Check sheet for the modelled part. Datum: model origin and axes. Units: mm. A direction names the side the tool comes from. Round coordinates to 2 decimals unless told otherwise and drop trailing zeros. Put each result on its own line as item: value.
```python
from build123d import *

# Parameters (mm, degrees)
F1_DEPTH       = 72.5
F3_D           = 5
F3_CBORE_D     = 10
F3_CBORE_DEPTH = 5
F4_R           = 2.5
F5_R           = 2.5


# Not quite as in the source:
# - ends of sketch curves that miss each other by under 0.0002 mm in the source are joined
# - the dataset's text gives a spline's control points without its knots; the knots are read off the source's solid


with BuildPart() as f1:
    # F0 (on Front) → F1 (new body)
    with BuildSketch(Plane.XZ):
        with BuildLine():
            add(Edge.make_bspline(
                [(-56.5881601574, 0.0419234738), (-55.5197950815, -0.7442946781), (-53.1301338185, -2.2933127374), (-48.9084685045, -4.5561843947), (-44.1859500973, -6.7339324001), (-39.1068883918, -8.7916644331), (-33.8193544964, -10.6897211609), (-29.3644227389, -12.1035605133), (-25.8455914341, -13.1126993817), (-22.383504382, -14.0327971877), (-19.4313477815, -14.7259719893), (-17.3706943762, -15.160741157), (-16.9593766332, -15.2455717325)],
                knots=[0, 0, 0, 0, 0.03125, 0.0625, 0.09375, 0.125, 0.15625, 0.1875, 0.203125, 0.21875, 0.25, 0.2578399244, 0.2578399244, 0.2578399244, 0.2578399244], degree=3))
            add(Edge.make_bspline(
                [(-56.5881601574, 0.0419234738), (-55.5355017666, 0.8486239051), (-53.1764131036, 2.443347048), (-48.9992069483, 4.7861572474), (-44.3187202519, 7.053077305), (-39.2793074327, 9.2063486815), (-34.0283660726, 11.2037109249), (-29.6007919855, 12.7012369201), (-26.1016179695, 13.7765699234), (-22.65755408, 14.761891198), (-19.6168305087, 15.5368665147), (-17.4672919643, 16.0305431026), (-16.9593493648, 16.1441983995)],
                knots=[1.43705e-05, 1.43705e-05, 1.43705e-05, 1.43705e-05, 0.03125, 0.0625, 0.09375, 0.125, 0.15625, 0.1875, 0.203125, 0.21875, 0.25, 0.2597438328, 0.2597438328, 0.2597438328, 0.2597438328], degree=3))
            Line((-16.9593493648, 16.1441983995), (-16.9593493648, 38.671177907))
            Line((-16.9593493648, 38.671177907), (-76.9551545382, 38.671177907))
            Line((-76.9551545382, 38.671177907), (-76.9551545382, -38.248822093))
            Line((-76.9551545382, -38.248822093), (-16.9593493648, -38.248822093))
            Line((-16.9593493648, -38.248822093), (-16.9593766332, -15.2455717325))
        make_face()
    extrude(amount=F1_DEPTH)

    # F3 (through all)
    with Locations(Plane(origin=(-76.9551545382, 0, 0), x_dir=(0, -1, 0), z_dir=(-1, 0, 0))):
        with Locations((10, 28.671177907), (62.5, 28.671177907), (62.5, -28.248822093), (10, -28.248822093)):
            CounterBoreHole(F3_D / 2, F3_CBORE_D / 2, F3_CBORE_DEPTH)

    # F4
    f4_edges = [f1.edges().sort_by_distance(p)[0] for p in [
        (-76.955155, -72.5, 0.211178),
        (-76.955155, -36.25, 38.671178),
        (-76.955155, 0, 0.211178),
        (-76.955155, -36.25, -38.248822),
    ]]
    fillet(f4_edges, radius=F4_R)

    # F5
    f5_edges = [f1.edges().sort_by_distance(p)[0] for p in [
        (-16.959349, -36.25, 38.671178),
        (-16.959349, -72.5, 27.407688),
        (-16.959349, 0, 27.407688),
        (-16.959363, 0, -26.747197),
        (-16.959349, -36.25, -38.248822),
        (-16.959363, -72.5, -26.747197),
    ]]
    fillet(f5_edges, radius=F5_R)


solid = f1.part
```
Item 1: Release check for a two-part mould opening along Z. For faces 3 (the flat face through (-47, -36, -38.249)), 4 (the cylindrical face through (-76.24, -36.76, 37.92)), 5 (the cylindrical face through (-74.49, -58.53, 25.63)), 6 (the flat face through (-47, 0, 9)) record: +Z half, -Z half, draft (parallel to the pull), parting line (faces both ways), or undercut.
Filled sheet:
face 3: -Z half
face 4: +Z half
face 5: undercut
face 6: draft
Item 2: Tool access check on faces 1 (the flat face through (-71.955, -12, -30)), 2 (the flat face through (-16.959, -36, 26)). Record the directions out of +Z, -Z, +X, -X, +Y, -Y that give a thin tool (end or side, any length) a straight path to the whole face; none if there is none.
Filled sheet:
face 1: -X
face 2: +Z, -Z, +X, +Y, -Y
Item 3: Thickness scan on line 1 (Z direction, x = -73.8, y = -10); line 2 (Y direction, x = -59, z = 29); line 3 (Z direction, x = -55, y = -10). Record the ranges inside material, lowest first. Write a range as from..to.
Filled sheet:
line 1: -38.25..-33.25, -23.25..23.67, 33.67..38.67
line 2: -72.5..-64.98, -60.02..-12.48, -7.52..0
line 3: -38.25..-30.75, -25.75..-1.06, 1.19..26.17, 31.17..38.67
Item 4: Section check A-A on x = -21. Count the separate pieces of the cut face and the enclosed holes in it, then the cut area to 3 significant figures.
Filled sheet:
separate pieces: 2
enclosed holes: 4
area: 3,360 mm²
Item 5: Go/stop test with flat-tipped pins: pin 1 (8 mm diameter, centred on y = -62.5, z = -28.25, fed in from -X); pin 2 (4 mm diameter, centred on y = -62.5, z = 28.67, fed in from +X). Record where each tip stops, or that it passes through.
Filled sheet:
pin 1: x = -71.96
pin 2: through
